The model under review builds one solid part; all positions refer to its coordinate system, in mm. A direction names the side the tool comes from. Coordinates: 2 decimals unless noted, no trailing zeros. Order: outer loops, then holes, each group sorted by start corner. A loop starts at its lowest first (then second) coordinate and runs counter-clockwise, first axis right, second up.
Autodesk Inventor part; units mm, degrees
ref_plane "YZ Plane" through (0, 0, 0) normal (1, 0, 0) x (0, 1, 0)
ref_plane "XZ Plane" through (0, 0, 0) normal (0, 1, 0) x (-1, 0, 0)
ref_plane "XY Plane" through (0, 0, 0) normal (0, 0, 1) x (1, 0, 0)
sketch "スケッチ1" plane through (0, 0, 0) normal (1, 0, 0) x (0, 1, 0)
  line L0 (24, 0) -> (24, -2)
  line L1 (24, -2) -> (26, -2)
  line L2 (26, -2) -> (26, -9)
  line L3 (26, -9) -> (37.5, -9)
  line L4 (37.5, -9) -> (37.5, 0)
  line L5 (37.5, 0) -> (24, 0)
  line L6 (0, -10.8) -> (0, 1.8)
  point P0 (0, 0)
  dimension "d0" = 26
  dimension "d1" = 37.5
  dimension "d2" = 7
  dimension "d3" = 2
  dimension "d4" = 2
revolve "回転1" add sketch "スケッチ1" angle 360 about axis through (0, 0, -10) along (0, 0, 1)
sketch "スケッチ2" plane through (0, 0, -9) normal (0, 0, -1) x (-1, 0, 0)
  circle A0 centre (0, 0) radius 32
  point P0 (0, 32)
  point P1 (-27.7128, 16)
  point P2 (-27.7128, -16)
  point P3 (0, -32)
  point P4 (27.7128, -16)
  point P5 (27.7128, 16)
  dimension "d6" = 64
  dimension "d9" = 360
hole "穴1" at (0, 32, -9) at (27.7128, 16, -9) at (27.7128, -16, -9) at (0, -32, -9) at (-27.7128, -16, -9) at (-27.7128, 16, -9) direction (0, 0, 1) diameter 4.5 end through all
sketch "スケッチ3" plane through (0, 0, -9) normal (0, 0, -1) x (-1, 0, 0)
  circle A0 centre (-37.5, 0) radius 4.8
  circle A1 centre (0, 0) radius 37.5
  point P0 (-37.1928, 4.7902)
  point P1 (-37.1928, -4.7902)
  dimension "d18" = 9.6
extrude "押し出し1" add sketch "スケッチ3" against normal blind 5 contours A1 A0 picked at (-39.0772, 0)
fillet "フィレット1" radius 4 2 edges at (37.1928, 4.7902, -6.5) (37.1928, -4.7902, -6.5)
properties part number "unit-base1" material "ABS プラスチック"
(1) We need section D-D, the plane y = -32. Write out the cut boundary in (x, z), and give its area (3 significant figures).
A:
outline: (-19.55, -9) - (-2.25, -9) - (-2.25, 0) - (-19.55, 0) - close; (2.25, -9) - (19.55, -9) - (19.55, 0) - (2.25, 0) - close
area: 311 mm2
(2) We need section B-B, the plane x = 8. Write out the cut boundary in (y, z), and give its area (3 significant figures).
A:
outline: (-36.64, -9) - (-24.74, -9) - (-24.74, -2) - (-22.63, -2) - (-22.63, 0) - (-36.64, 0) - close; (22.63, -2) - (24.74, -2) - (24.74, -9) - (36.64, -9) - (36.64, 0) - (22.63, 0) - close
area: 223 mm2
(3) Draft analysis for pull direction Y (two halves, no side actions). For faces 1 (the face through (-37.18, -4.88, -4.44)), 2 (the face through (40, 0, -4)), 3 (the face through (0.86, 34.08, -4.44)), state which applies: released by +Y, released by -Y, zero draft, split by the parting line, or undercut.
A:
face 1: split by the parting line
face 2: zero draft
face 3: undercut
(4) For pin 1 Ø3 at (y, z) = (-28, -4) entering from +X; pin 2 Ø7 at (x, y) = (0, -32) entering from +Z; pin 3 Ø5 at (x, z) = (-27.5, -3) entering from -Y; pin 4 Ø3 at (y, z) = (-23.5, -6.5) entering from -X, all flat-tipped, find the tip position at first contact; note any pin that passes through.
A:
pin 1: stops at x = 26.53
pin 2: stops at z = 0
pin 3: stops at y = -27.95
pin 4: stops at x = -30.37
(5) We need section A-A, the plane y = 0. Write out the cut boundary in (x, z), and give its area (3 significant figures).
A:
outline: (-37.5, -9) - (-26, -9) - (-26, -2) - (-24, -2) - (-24, 0) - (-37.5, 0) - close; (24, -2) - (26, -2) - (26, -9) - (42.3, -9) - (42.3, -4) - (37.5, -4) - (37.5, 0) - (24, 0) - close
area: 239 mm2
(6) We need section C-C, the plane y = 16. Write out the cut boundary in (x, z), and give its area (3 significant figures).
A:
outline: (-33.92, -9) - (-29.96, -9) - (-29.96, 0) - (-33.92, 0) - close; (-25.46, -9) - (-20.49, -9) - (-20.49, -2) - (-17.89, -2) - (-17.89, 0) - (-25.46, 0) - close; (17.89, -2) - (20.49, -2) - (20.49, -9) - (25.46, -9) - (25.46, 0) - (17.89, 0) - close; (29.96, -9) - (33.92, -9) - (33.92, 0) - (29.96, 0) - close
area: 171 mm2
(7) Wall thickness on probe 1 along Y at (x, z) = (0, -6.25); probe 2 along X at (y, z) = (15.5, -8); probe 3 along X at (y, z) = (32, -3.25): over which ranges is each line inside the solid? List them lowest first.
A:
probe 1: y = -37.5 to -34.25, -29.75 to -26, 26 to 29.75, 34.25 to 37.5
probe 2: x = -34.15 to -29.91, -25.52 to -20.87, 20.87 to 25.52, 29.91 to 34.15
probe 3: x = -19.55 to -2.25, 2.25 to 19.55
(8) Machinability: for faces 4 (the face through (-15.821, -20.633, -5.549)), 5 (the face through (-0.676, -29.854, -4.437)), which of the approach directions +Z, -Z, +X, -X, +Y, -Y give a long, thin tool a straight path to every point of the face, cutting with its end or side? Answer none if there is none.
A:
face 4: -Z
face 5: +Z, -Z
